Answer from the drawing. Dimensions are ordinates in mm from the lowest x, y and z of the part. A direction names the side the tool comes from. Round coordinates to 2 decimals unless told otherwise and drop trailing zeros. Write each loop counter-clockwise with the first axis right and the second up, starting at its lowest first coordinate (ties: lowest second). Pieces come first, ordered by that corner, then holes. Notation, with made-up numbers: (-6, 13) -> (25, 13) arc R32 cw to (25, 41) -> close; hole circle Ø10 at (67.25, 47.5). An arc over 180 degrees is marked (long way). Return JSON: item names as keys, results as strings. Group by question number.
(1) The mould has two halves that part along X. Classify the marked faces 1, 2, 3 and 4: released by +X, released by -X, zero draft, split by the parting line, or undercut.
(2) For the marked faces 5 and 6, determine the directions among +Z, -Z, +X, -X, +Y, -Y from which every point of the face is accessible in a straight line to the end or side of a thin tool.
(3) A cutting plane is placed at B-B on y = 1.75. Give the vertices of the cut face in (x, z), then the cut area to 3 significant figures.
(4) A cutting plane is placed at D-D on y = 19.75. Give the vertices of the cut face in (x, z).
(5) A cutting plane is placed at A-A on x = 30. Give the vertices of the cut face in (y, z).
(6) Straight lines are drawn through the part: line 1 (Z direction, x = 30, y = 3.1); line 2 (Z direction, x = 49, y = 17); line 3 (X direction, y = 3, z = 10.25). For each, find the intervals that lie inside material, in ascending order.
(7) Given pin 1 (2.5 mm diameter, centred on x = 49, z = 25, fed in from +Y); pin 2 (9 mm diameter, centred on x = 30, z = 20, fed in from -Y); pin 3 (6.5 mm diameter, centred on y = 20, z = 10, fed in from -X); pin 4 (2 mm diameter, centred on x = 15.5, y = 15.5, fed in from +Z) (1 decimal), each flat-ended and moving along its own axis, determine where each tip first touches the part or whether it passes through.
(8) A cutting plane is placed at C-C on z = 21. Give the vertices of the cut face in (x, y).
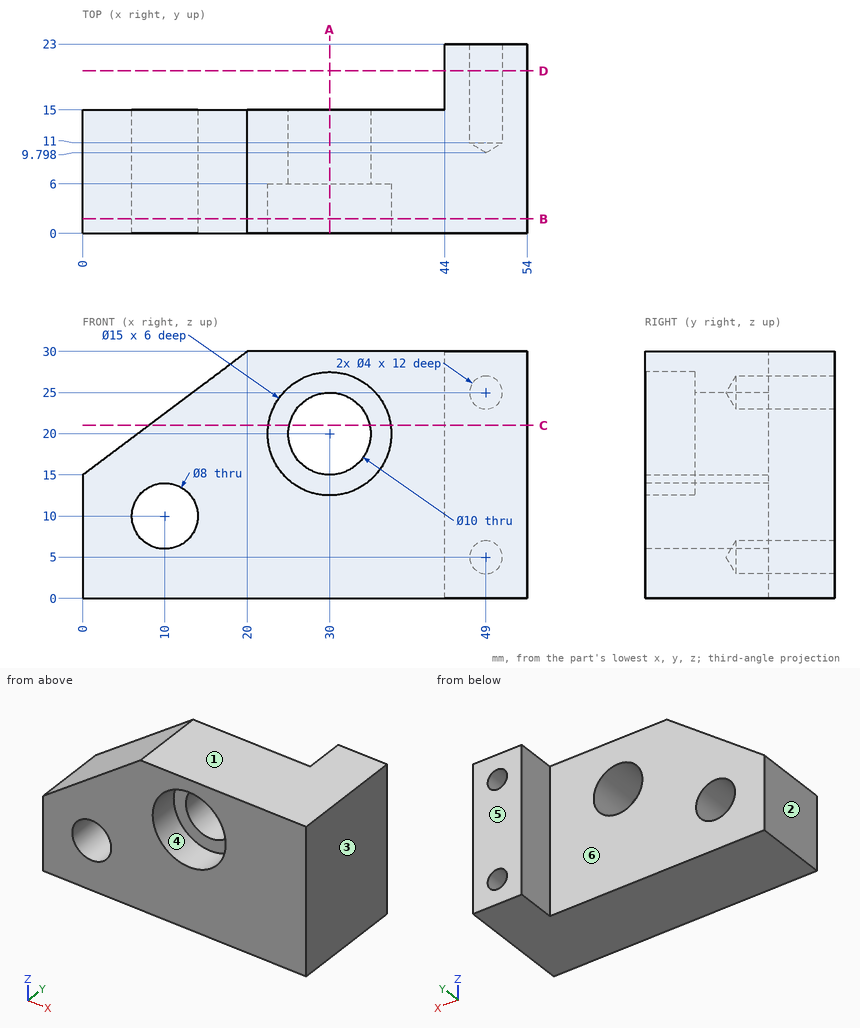
Checks:
{
 "1": {"face 1": "zero draft", "face 2": "released by -X", "face 3": "released by +X", "face 4": "undercut"},
 "2": {"face 5": "+Z, -Z, +X, -X, +Y", "face 6": "+Z, -Z, -X, +Y"},
 "3": {"outline": "(0, 0) -> (54, 0) -> (54, 30) -> (20, 30) -> (0, 15) -> close; hole circle Ø8 at (10, 10); hole circle Ø15 at (30, 20)", "area": "1,240 mm^2"},
 "4": {"outline": "(44, 0) -> (54, 0) -> (54, 30) -> (44, 30) -> close; hole circle Ø4 at (49, 5); hole circle Ø4 at (49, 25)"},
 "5": {"outline": "(0, 0) -> (15, 0) -> (15, 15) -> (6, 15) -> (6, 12.5) -> (0, 12.5) -> close; (0, 27.5) -> (6, 27.5) -> (6, 25) -> (15, 25) -> (15, 30) -> (0, 30) -> close"},
 "6": {"line 1": "z = 0 to 12.5, 27.5 to 30", "line 2": "z = 0 to 3, 7 to 23, 27 to 30", "line 3": "x = 0 to 6.01, 13.99 to 54"},
 "7": {"pin 1": "stops at y = 10.55", "pin 2": "passes through", "pin 3": "stops at x = 44", "pin 4": "stops at z = 27.3"},
 "8": {"outline": "(8, 0) -> (22.57, 0) -> (22.57, 6) -> (25.1, 6) -> (25.1, 15) -> (8, 15) -> close; (34.9, 6) -> (37.43, 6) -> (37.43, 0) -> (54, 0) -> (54, 23) -> (44, 23) -> (44, 15) -> (34.9, 15) -> close"}
}
